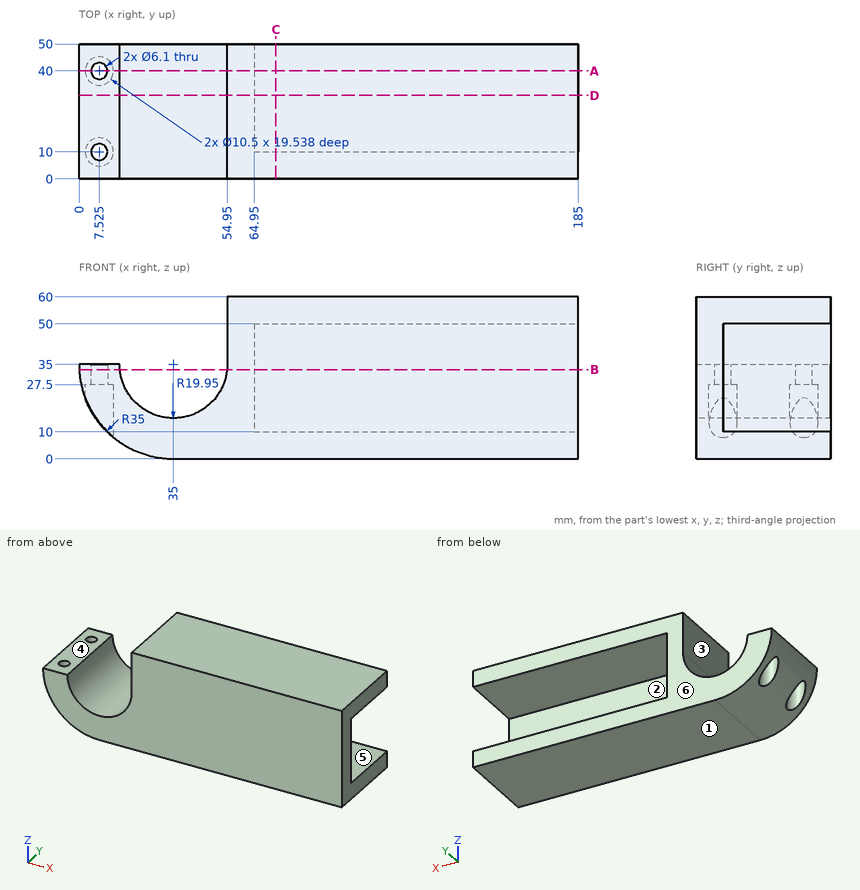
For this review, use the dimensioned drawing (mm, ordinates from the lowest corner) and the shaded views. A direction names the side the tool comes from. Coordinates: 2 decimals unless noted, no trailing zeros. Loops run counter-clockwise (first coordinate to the right, second up) from the corner with the lowest first, then second, coordinate; pieces in that order, holes last. Notation, with made-up numbers: (-2, -15.5) - (9, -15.5) arc R33 cw to (9, 20.5) - close; hole circle Ø7 at (-19, -14.5). An arc over 180 degrees is marked (long way). Use one line per item in the form item = value. Start each with the question number.
1) To check wall thickness, follow probe 1 along Z at (x, y) = (128, 32); probe 2 along X at (y, z) = (5.5, 24.5); probe 3 along Y at (x, z) = (110.5, 36). State the ranges of each line that lie inside material, in increasing order. Write a range as from..to.
2) Take a section at B-B (z = 33). State how many separate pieces and enclosed holes the cut face has, plus the area to 3 significant figures.
3) Take a section at C-C (x = 73). State the section outline as (y, z) points.
4) For the marked faces 1, 2 and 3, list the 3-axis set-ups (+Z, -Z, +X, -X, +Y, -Y) from which the entire face can be reached by the end or side of a thin tool; tool diameter is ignored.
5) Take a section at A-A (y = 40). State the section outline as (x, z) points (3 decimals).
6) For pin 1 (16.5 mm diameter, centred on x = 9, y = 37, fed in from +Z); pin 2 (12 mm diameter, centred on y = 37, z = 17, fed in from +X); pin 3 (8.5 mm diameter, centred on x = 7.525, y = 40, fed in from -Z), all flat-tipped, find the tip position at first contact; note any pin that passes through.
7) Take a section at D-D (y = 31). State the section outline as (x, z) points, plus the area to 3 significant figures.
8) Draft analysis for pull direction Z (two halves, no side actions). For the marked faces 4, 5 and 6, state which applies: released by +Z, released by -Z, zero draft, split by the parting line, or undercut.
From the geometry:
q1.probe_1 = 0..10, 50..60
q1.probe_2 = 1.61..4.82, 10.23..18.04, 51.96..185
q1.probe_3 = 0..10
q2.separate_pieces = 2
q2.enclosed_holes = 2
q2.area = 2,400 mm2
q3.outline = (0, 0) - (50, 0) - (50, 10) - (10, 10) - (10, 50) - (50, 50) - (50, 60) - (0, 60) - close
q4.face_1 = -Z, +X, -X, +Y, -Y
q4.face_2 = +X, +Y
q4.face_3 = +Z, -X, +Y, -Y
q5.outline = (0, 35) arc R35 ccw to (2.275, 22.587) - (2.275, 27.5) - (4.475, 27.5) - (4.475, 35) - close; (10.575, 27.5) - (12.775, 27.5) - (12.775, 7.962) arc R35 ccw to (35, 0) - (185, 0) - (185, 10) - (64.95, 10) - (64.95, 50) - (185, 50) - (185, 60) - (54.95, 60) - (54.95, 35) arc R19.95 cw to (15.05, 35) - (10.575, 35) - close
q6.pin_1 = 35
q6.pin_2 = 64.95
q6.pin_3 = 27.5
q7.outline = (0, 35) arc R35 ccw to (35, 0) - (185, 0) - (185, 10) - (64.95, 10) - (64.95, 50) - (185, 50) - (185, 60) - (54.95, 60) - (54.95, 35) arc R19.95 cw to (15.05, 35) - close
q7.area = 4,040 mm2
q8.face_4 = released by +Z
q8.face_5 = undercut
q8.face_6 = zero draft
